Geometry: see drawing. Coordinates: mm, zero at the bounding-box minimum. Round coordinates to 2 decimals unless told otherwise and drop trailing zeros. Write each loop counter-clockwise with the first axis right and the second up, starting at its lowest first coordinate (ties: lowest second). Pieces come first, ordered by that corner, then holes. Notation, with made-up numbers: M 56,10 L 94,10 A36 cw 94,45 Z; hole C 31,40 d3. An arc over 180 degrees is marked long. Use a Markdown table: item, result.
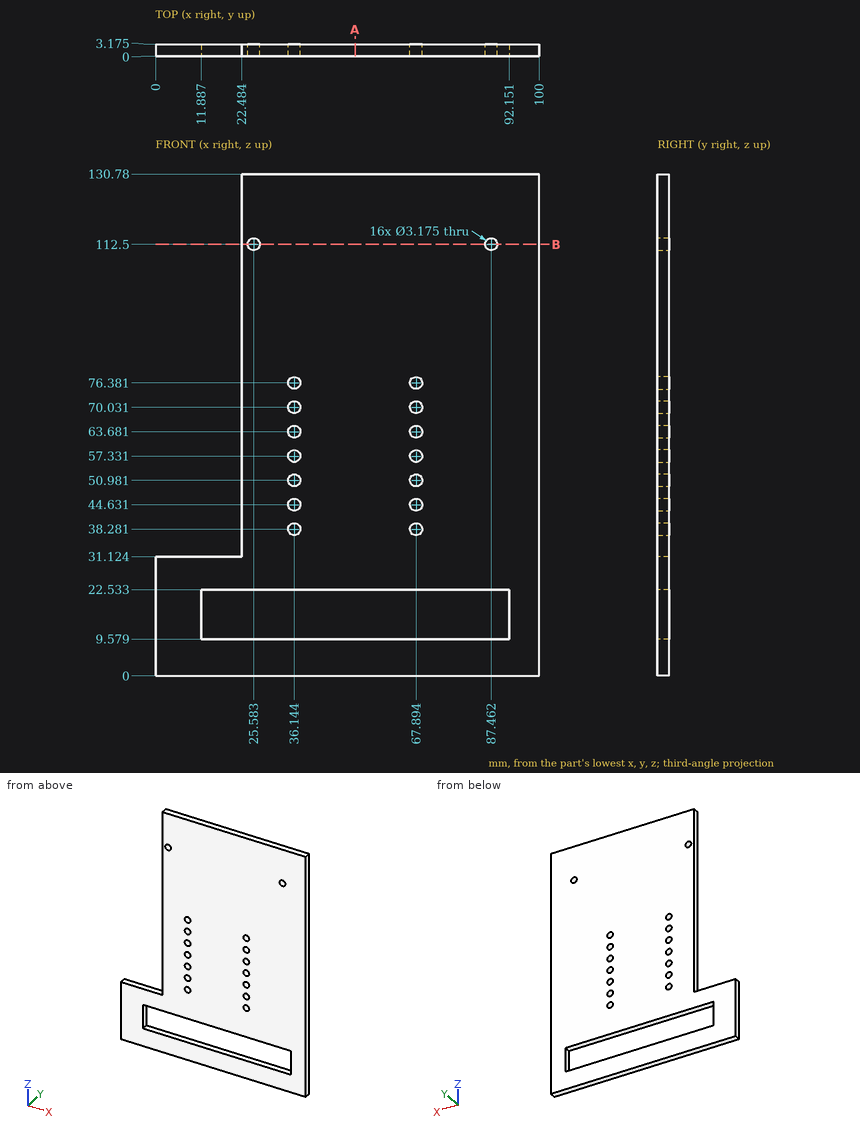
Q1. Section B-B on z = 112.5. Give the number of separate pieces and of enclosed holes in the cut face, plus the area to 3 significant figures.
Results are:
| item | result |
|---|---|
| separate pieces | 3 |
| enclosed holes | 0 |
| area | 226 mm^2 |
Q2. Section A-A on x = 52. Return loops of the section in (y, z) (1 decimal), plus the area to 3 significant figures.
Results are:
| item | result |
|---|---|
| outline | M 0,0 L 3.2,0 L 3.2,9.6 L 0,9.6 Z; M 0,22.5 L 3.2,22.5 L 3.2,130.8 L 0,130.8 Z |
| area | 374 mm^2 |
Q3. Line query: L1, parallel to X at y = 2.6, z = 57.5 (1 decimal); L2, parallel to Z at x = 17, y = 1.2 (1 decimal); L3, parallel to Z at x = 88.5, y = 2.3 (1 decimal). Output: solid intervals per line, ascending.
Results are:
| item | result |
|---|---|
| L1 | 22.5 to 34.6, 37.7 to 66.3, 69.5 to 100 |
| L2 | 0 to 9.6, 22.5 to 31.1 |
| L3 | 0 to 9.6, 22.5 to 111.3, 113.7 to 130.8 |
Q4. First-contact query: pin 1 Ø2.5 at (x, z) = (36.14, 57.33) entering from -Y; pin 2 Ø1 at (y, z) = (1, 88) entering from -X. Flat tips, straight axial feed; report the tip coordinate or a pass-through.
Results are:
| item | result |
|---|---|
| pin 1 | through |
| pin 2 | x = 22.48 |
